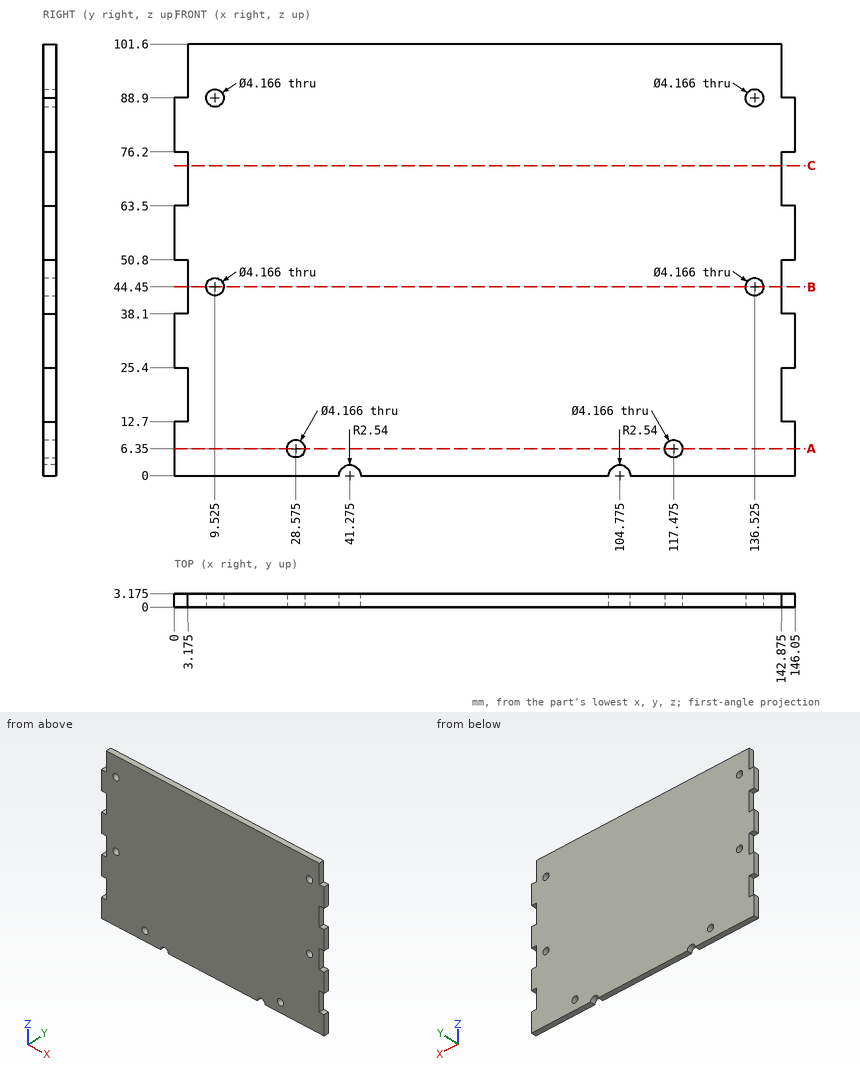
The figure shows three views and two pictorial views of one solid part (mm, origin at its lowest corner). Answer the questions. Give positions to 0.01 mm unless a question says otherwise; leave off trailing zeros. Order: outer loops, then holes, each group sorted by start corner. A loop starts at its lowest first (then second) coordinate and runs counter-clockwise, first axis right, second up. Notation, with made-up numbers: (15.25, 69) -> (22.25, 69) arc R14 ccw to (22.25, 82) -> close; hole circle Ø9 at (-34.75, -14). An arc over 180 degrees is marked (long way). Answer as a JSON object with one key per item and string values. Group by question number.
Item 1: The part is cut by section A-A on z = 6.35. Give the number of separate pieces and of enclosed holes in the cut face, and give its area (3 significant figures).
Item 2: The part is cut by section B-B on z = 44.45. Write down the section's boundary in (x, y) (1 decimal).
Item 3: The part is cut by section C-C on z = 73. Write down the section's boundary in (x, y) (1 decimal).
Item 4: Flat-ended cylindrical pins translate along their axes: pin 1 (1 mm diameter, centred on y = 1.5, z = 95, fed in from +X) (3 decimals); pin 2 (1 mm diameter, centred on x = 144, y = 1.5, fed in from +Z). Find the tip coordinate at first contact, or state that the pin passes through.
Item 5: Consider L1, parallel to X at y = 1.35, z = 44.45 (1 decimal); L2, parallel to X at y = 0.7, z = 6.35; L3, parallel to Z at x = 28.5, y = 1.7. Determine where each line is inside the solid, lowest interval first. Write a range as from..to.
Result set:
{
 "1": {"separate pieces": "3", "enclosed holes": "0", "area": "437 mm²"},
 "2": {"outline": "(3.2, 0) -> (7.4, 0) -> (7.4, 3.2) -> (3.2, 3.2) -> close; (11.6, 0) -> (134.4, 0) -> (134.4, 3.2) -> (11.6, 3.2) -> close; (138.6, 0) -> (142.9, 0) -> (142.9, 3.2) -> (138.6, 3.2) -> close"},
 "3": {"outline": "(3.2, 0) -> (142.9, 0) -> (142.9, 3.2) -> (3.2, 3.2) -> close"},
 "4": {"pin 1": "x = 142.875", "pin 2": "z = 88.9"},
 "5": {"L1": "3.2..7.4, 11.6..134.4, 138.6..142.9", "L2": "0..26.49, 30.66..115.39, 119.56..146.05", "L3": "0..4.27, 8.43..101.6"}
}
